from build123d import *

# Parameters (mm, degrees)
SKETCH001_W      = 20
SKETCH001_H      = 450
EXTRUDE001_DEPTH = 850
SKETCH_W         = 2430
SKETCH_H         = 450
EXTRUDE_DEPTH    = 20


with BuildPart() as obj1:
    # Sketch001 → Extrude001 (new body)
    with BuildSketch(Plane.XY):
        with Locations((10, 225)):
            Rectangle(SKETCH001_W, SKETCH001_H)
    extrude(amount=EXTRUDE001_DEPTH)


with BuildPart() as obj2:
    # Clone001 base: copy of obj1
    add(obj1.part)


with BuildPart() as obj2_1:
    # Clone001 placement: moved
    add(obj2.part.moved(Location((2450, 0, 0))))


with BuildPart() as tampo_inferior:
    # Sketch → Extrude (new body)
    with BuildSketch(Plane.XY):
        with Locations((1215, 225)):
            Rectangle(SKETCH_W, SKETCH_H)
    extrude(amount=EXTRUDE_DEPTH)


with BuildPart() as tampo_inferior_1:
    # Extrude placement: moved
    add(tampo_inferior.part.moved(Location((20, 0, 0))))


with BuildPart() as tampo:
    # Clone base: copy of Tampo inferior
    add(tampo_inferior_1.part)


with BuildPart() as tampo_1:
    # Clone placement: moved
    add(tampo.part.moved(Location((0, 0, 830))))


with BuildPart() as obj3:
    # Fusion base: copy of Tampo inferior
    add(tampo_inferior_1.part)

    # Fusion: union obj2, tampo, obj1
    add(obj2_1.part)
    add(tampo_1.part)
    add(obj1.part)


solid = obj3.part
Verification items for the finished model (mm, model axes). A direction names the side the tool comes from. Coordinates: 2 decimals unless noted, no trailing zeros. Order: outer loops, then holes, each group sorted by start corner. A loop starts at its lowest first (then second) coordinate and runs counter-clockwise, first axis right, second up. Notation, with made-up numbers: M 8,-18.5 L 51,-18.5 A11 cw 51,-4.5 Z; hole C 82.25,43 d5. An arc over 180 degrees is marked long. One line per item, written item: value. Start each with the question number.
Item 1: Mould release check, pull along X, two halves, no side actions. Record for faces 1 (the flat face through (1218, 228, 850)), 2 (the flat face through (2450, 222, 419)), 3 (the flat face through (2470, 222, 419)): pulls with the +X half, pulls with the -X half, needs draft (parallel to the pull), parting line crosses it, or undercut.
Item 2: Sectioned sample at C-C on y = 196. Record the cut outline in (x, z).
Item 3: Access from +Z, -Z, +X, -X, +Y, -Y to the whole of each face (thin tool, end or side, straight path). Record for faces 4 (the flat face through (20, 222, 419)), 5 (the flat face through (1229, 0, 14)).
Item 4: Sectioned sample at B-B on x = 845.5. Record the cut outline in (y, z).
Item 5: Thickness scan on probe 1 along Z at (x, y) = (983.5, 350); probe 2 along X at (y, z) = (403.5, 100). Record the ranges inside material, lowest first.
Item 6: Sectioned sample at A-A on z = 358.5. Record the cut outline in (x, y), then the cut area to 3 significant figures.
Calculated:
1. face 1: needs draft
1. face 2: undercut
1. face 3: pulls with the +X half
2. outline: M 0,0 L 2470,0 L 2470,850 L 0,850 Z; hole M 20,20 L 2450,20 L 2450,830 L 20,830 Z
3. face 4: +Y, -Y
3. face 5: +Z, -Z, +X, -X, -Y
4. outline: M 0,0 L 450,0 L 450,20 L 0,20 Z; M 0,830 L 450,830 L 450,850 L 0,850 Z
5. probe 1: 0 to 20, 830 to 850
5. probe 2: 0 to 20, 2450 to 2470
6. outline: M 0,0 L 20,0 L 20,450 L 0,450 Z; M 2450,0 L 2470,0 L 2470,450 L 2450,450 Z
6. area: 18,000 mm^2
